Can you work these out from the model? Positions are in its coordinate system, mm. Coordinates: 2 decimals unless noted, no trailing zeros. Loops run counter-clockwise (first coordinate to the right, second up) from the corner with the lowest first, then second, coordinate; pieces in that order, holes last.
```python
from build123d import *

# Parameters (mm, degrees)
SKETCH1_W           = 211
SKETCH1_H           = 75
BOSS_EXTRUDE1_DEPTH = 1.5
BOSS_EXTRUDE2_DEPTH = 1.5


with BuildPart() as part:
    # Sketch1 → Boss-Extrude1 (new body)
    with BuildSketch(Plane.XY):
        with Locations((105.5, -37.5)):
            Rectangle(SKETCH1_W, SKETCH1_H)
    extrude(amount=BOSS_EXTRUDE1_DEPTH)

    # Sketch2 → Boss-Extrude2 (add)
    with BuildSketch(Plane.XY):
        Polygon((0, 0), (0, 140), (15, 140), (42.712812921, 124), (75, 68.076951546), (75, 0), align=None)
    extrude(amount=BOSS_EXTRUDE2_DEPTH)


solid = part.part
```
(1) If I drill on probe 1 along Y at (x, z) = (195, 1.2); probe 2 along X at (y, z) = (13, 1.45); probe 3 along Y at (x, z) = (17, 0.35), over which ranges is the centre line in solid material (lowest first)?
Check values:
probe 1: y = -75 to 0
probe 2: x = 0 to 75
probe 3: y = -75 to 138.85
(2) I want a section at B-B on x = 131.5. Write out the boundary of the cut face in (y, z).
Check values:
outline: (-75, 0) - (0, 0) - (0, 1.5) - (-75, 1.5) - close
(3) I want a section at A-A on z = 0.8. Write out the boundary of the cut face in (x, y).
Check values:
outline: (0, -75) - (211, -75) - (211, 0) - (75, 0) - (75, 68.08) - (42.71, 124) - (15, 140) - (0, 140) - close
(4) I want a section at C-C on y = 30.5. Write out the boundary of the cut face in (x, z), then the cut area to 4 significant figures.
Check values:
outline: (0, 0) - (75, 0) - (75, 1.5) - (0, 1.5) - close
area: 112.5 mm2
